Work out the finished part from the listing and answer in its coordinate system (mm). A direction names the side the tool comes from. Round coordinates to 2 decimals unless told otherwise and drop trailing zeros. Order: outer loops, then holes, each group sorted by start corner. A loop starts at its lowest first (then second) coordinate and runs counter-clockwise, first axis right, second up. Notation, with made-up numbers: (-15, -16) - (6, -16) arc R18 ccw to (6, -3) - close; hole circle Ø9 at (10, 9). An arc over 180 degrees is marked (long way). Put each result on its own line as item: value.
```python
from build123d import *

# Parameters (mm, degrees)
F4_D           = 15
F4_CBORE_D     = 25.5
F4_CBORE_DEPTH = 16
F5_D           = 10.5
F6_D           = 16


with BuildPart() as f1:
    # F0 (on Front) → F1 (revolve)
    with BuildSketch(Plane.XZ):
        Polygon((30, -5), (30, 0), (80, 0), (80, 40), (33.075, 40), (33.075, 55), (0, 55), (0, 0), (0, -5), align=None)
    revolve(axis=Axis((0, 0, 27.5), (0, 0, -1)))

    # F4 (through all)
    with Locations(Plane.XY.offset(55)):
        with Locations((0, 0)):
            CounterBoreHole(F4_D / 2, F4_CBORE_D / 2, F4_CBORE_DEPTH)

    # F5 (through all)
    with Locations(Plane.XY.offset(40)):
        with Locations((-54.3528799063, 17.6603212285), (-33.5919271685, -46.2353212285), (33.5919271685, -46.2353212285), (54.3528799063, 17.6603212285)):
            Hole(F5_D / 2)

    # F6 (through all)
    with Locations(Plane.XY.offset(40)):
        with Locations((0, 57.15)):
            Hole(F6_D / 2)


solid = f1.part
```
1) A cutting plane is placed at A-A on x = 0. Write down the section's boundary in (y, z) (3 decimals).
Findings below:
outline: (-80, 0) - (-30, 0) - (-30, -5) - (-7.5, -5) - (-7.5, 39) - (-12.75, 39) - (-12.75, 55) - (-33.075, 55) - (-33.075, 40) - (-80, 40) - close; (7.5, -5) - (30, -5) - (30, 0) - (49.15, 0) - (49.15, 40) - (33.075, 40) - (33.075, 55) - (12.75, 55) - (12.75, 39) - (7.5, 39) - close; (65.15, 0) - (80, 0) - (80, 40) - (65.15, 40) - close
2) A cutting plane is placed at D-D on x = -64. Write down the section's boundary in (y, z).
Findings below:
outline: (-48, 0) - (48, 0) - (48, 40) - (-48, 40) - close
3) Straight lines are drawn through the part: L1, parallel to X at y = 0.5, z = 17; L2, parallel to Y at x = 0, z = 44.5 (3 decimals); L3, parallel to Z at x = 15.5, y = -70.5. For each, find the intervals that lie inside material, in ascending order. Write a range as from..to.
Findings below:
L1: x = -80..-7.48, 7.48..80
L2: y = -33.075..-12.75, 12.75..33.075
L3: z = 0..40
4) For faces 4 (the flat face through (-34, -1, 0)), 5 (the cylindrical face through (-2.764, -12.447, 47.112)), 6 (the flat face through (14, 0, 55)), determine the directions among +Z, -Z, +X, -X, +Y, -Y from which every point of the face is accessible in a straight line to the end or side of a thin tool.
Findings below:
face 4: -Z
face 5: +Z
face 6: +Z, +X, -X, +Y, -Y
5) Given pin 1 Ø13.5 at (x, y) = (-33.59, -46.24) entering from -Z; pin 2 Ø18.5 at (x, y) = (0, 57.15) entering from +Z; pin 3 Ø10 at (y, z) = (-4, 31) entering from -X; pin 4 Ø9.5 at (x, y) = (-54.35, 17.66) entering from -Z, each flat-ended and moving along its own axis, determine where each tip first touches the part or whether it passes through.
Findings below:
pin 1: stops at z = 0
pin 2: stops at z = 40
pin 3: stops at x = -80
pin 4: passes through
6) For a pull along X with two mould halves and no side action, classify faces 1 (the cylindrical face through (31.55, -9.93, 47.6)), 2 (the cylindrical face through (58.22, 21.21, 19.72)), 3 (the flat face through (34, -1, 40)) as pulls with the +X half, pulls with the -X half, needs draft (parallel to the pull), parting line crosses it, or undercut.
Findings below:
face 1: parting line crosses it
face 2: undercut
face 3: needs draft
7) A cutting plane is placed at C-C on z = 16. Write down the section's boundary in (x, y).
Findings below:
outline: circle Ø160 at (0, 0); hole circle Ø10.5 at (-54.35, 17.66); hole circle Ø10.5 at (-33.59, -46.24); hole circle Ø16 at (0, 57.15); hole circle Ø15 at (0, 0); hole circle Ø10.5 at (33.59, -46.24); hole circle Ø10.5 at (54.35, 17.66)
8) A cutting plane is placed at B-B on y = 0. Write down the section's boundary in (x, z) (3 decimals), then the cut area to 3 significant figures.
Findings below:
outline: (-80, 0) - (-30, 0) - (-30, -5) - (-7.5, -5) - (-7.5, 39) - (-12.75, 39) - (-12.75, 55) - (-33.075, 55) - (-33.075, 40) - (-80, 40) - close; (7.5, -5) - (30, -5) - (30, 0) - (80, 0) - (80, 40) - (33.075, 40) - (33.075, 55) - (12.75, 55) - (12.75, 39) - (7.5, 39) - close
area: 6,620 mm2
